from build123d import *

# Parameters (mm, degrees)
SKETCH2_W               = 1500
SKETCH2_H               = 150
BOSS_EXTRUDE1_DEPTH     = 600
SKETCH3_R               = 12.5
CUT_EXTRUDE2_DEPTH      = 250
MIRROR3_COPY_1_SKETCH_R = 12.5
MIRROR3_COPY_1_DEPTH    = 250
SKETCH4_R               = 12.5
CUT_EXTRUDE3_DEPTH      = 50
SKETCH5_W               = 1020
SKETCH5_H               = 1050
CUT_EXTRUDE4_DEPTH      = 100
FILLET1_R               = 20


with BuildPart() as part:
    # Sketch2 → Boss-Extrude1 (new body, symmetric)
    with BuildSketch(Plane.XY):
        Rectangle(SKETCH2_W, SKETCH2_H)
    extrude(amount=BOSS_EXTRUDE1_DEPTH, both=True)

    # Sketch3 → Cut-Extrude2 (cut)
    with BuildSketch(Plane.XY.offset(600)):
        with Locations((-600, -25)):
            Circle(SKETCH3_R)
    cut_extrude2 = extrude(amount=-CUT_EXTRUDE2_DEPTH, mode=Mode.SUBTRACT)

    # Mirror2: Cut-Extrude2 across plane
    add(cut_extrude2.mirror(Plane(origin=(0, 0, 0), x_dir=(0, 0, 1), z_dir=(1, 0, 0))), mode=Mode.SUBTRACT)

    # Mirror3: Cut-Extrude2 across plane
    add(cut_extrude2.mirror(Plane.XY), mode=Mode.SUBTRACT)

    # Mirror3 copy 1 sketch → Mirror3 copy 1 (cut)
    with BuildSketch(Plane(origin=(0, 0, -600), x_dir=(-1, 0, 0), z_dir=(0, 0, -1))):
        with Locations((-600, -25)):
            Circle(MIRROR3_COPY_1_SKETCH_R)
    extrude(amount=-MIRROR3_COPY_1_DEPTH, mode=Mode.SUBTRACT)

    # Sketch4 → Cut-Extrude3 (cut)
    with BuildSketch(Plane(origin=(0, 75, 0), x_dir=(1, 0, 0), z_dir=(0, 1, 0))):
        with Locations((-650, 0)):
            Circle(SKETCH4_R)
    extrude(amount=-CUT_EXTRUDE3_DEPTH, mode=Mode.SUBTRACT)

    # Sketch5 → Cut-Extrude4 (cut)
    with BuildSketch(Plane(origin=(0, 75, 0), x_dir=(1, 0, 0), z_dir=(0, 1, 0))):
        Rectangle(SKETCH5_W, SKETCH5_H)
    extrude(amount=-CUT_EXTRUDE4_DEPTH, mode=Mode.SUBTRACT)

    # Fillet1
    fillet1_edges = [part.edges().sort_by_distance(p)[0] for p in [
        (-750, 0, 600),
        (0, -75, 600),
        (510, -25, 0),
        (510, 25, -525),
        (0, -25, 525),
        (510, 25, 525),
        (-510, -25, 0),
        (-510, 25, 525),
        (0, -25, -525),
        (-510, 25, -525),
        (510, 75, 0),
        (0, 75, -525),
        (-510, 75, 0),
        (0, 75, 525),
        (750, 0, 600),
        (0, -75, -600),
        (-750, 0, -600),
        (750, 0, -600),
        (750, -75, 0),
        (-750, -75, 0),
    ]]
    fillet(fillet1_edges, radius=FILLET1_R)


solid = part.part
Can you work these out from the model? Positions are in its coordinate system, mm. A direction names the side the tool comes from. Coordinates: 2 decimals unless noted, no trailing zeros. Write each loop counter-clockwise with the first axis right and the second up, starting at its lowest first coordinate (ties: lowest second). Pieces come first, ordered by that corner, then holes. Notation, with made-up numbers: (87, 80) -> (99, 80) arc R7 ccw to (99, 92) -> close; hole circle Ø7 at (17, -37). An arc over 180 degrees is marked (long way). Answer as CSV lines item,"result".
1) On a 3-axis mill with a long thin cutter (end or side, diameter ignored), from which of +Z, -Z, +X, -X, +Y, -Y can I reach the whole of each face in a straight line? I mean faces 5 (the flat face through (-10, 11, -600)), 6 (the flat face through (510, 25, 7)). Say none if no direction works.
Check result:
face 5,"-Z, +X, -X, +Y, -Y"
face 6,"+Y"
2) If we section it at B-B on x = -189: Please give me the cut outline in (y, z).
Check result:
outline,"(-75, -580) arc R20 ccw to (-55, -600) -> (75, -600) -> (75, -545) arc R20 ccw to (55, -525) -> (-5, -525) arc R20 cw to (-25, -505) -> (-25, 505) arc R20 cw to (-5, 525) -> (55, 525) arc R20 ccw to (75, 545) -> (75, 600) -> (-55, 600) arc R20 ccw to (-75, 580) -> close"
3) If we mould it in two halves opening along X, with no side actions, what happens to faces 1 (the flat face through (-510, 25, 7)), 2 (the flat face through (-7, 25, -525)), 3 (the flat face through (-10, -75, 8)), 4 (the flat face through (750, 9, 8))? For each: +X half, -X half, draft (parallel to the pull), parting line (faces both ways), or undercut.
Check result:
face 1,"undercut"
face 2,"undercut"
face 3,"draft"
face 4,"+X half"
4) Will these pins go through, and if not, where does the flat tip stop? P1, Ø7.5, axis at x = -601, y = -27, coming from the +Z side; P2, Ø12, axis at x = 244, z = 363.5, coming from the +Y side; P3, Ø15, axis at x = 600, y = -25, coming from the -Z side.
Check result:
P1,"z = 350"
P2,"y = -25"
P3,"z = -350"
5) If we section it at A-A on z = -369.5: Please give me the cut outline in (x, y), then the cut area to 3 significant figures.
Check result:
outline,"(-750, -55) arc R20 ccw to (-730, -75) -> (730, -75) arc R20 ccw to (750, -55) -> (750, 75) -> (530, 75) arc R20 ccw to (510, 55) -> (510, -5) arc R20 cw to (490, -25) -> (-490, -25) arc R20 cw to (-510, -5) -> (-510, 55) arc R20 ccw to (-530, 75) -> (-750, 75) -> close; hole circle Ø25 at (-600, -25); hole circle Ø25 at (600, -25)"
area,"122,000 mm²"
6) If we section it at C-C on z = -77.5: Please give me the cut outline in (x, y), then the cut area to 3 significant figures.
Check result:
outline,"(-750, -55) arc R20 ccw to (-730, -75) -> (730, -75) arc R20 ccw to (750, -55) -> (750, 75) -> (530, 75) arc R20 ccw to (510, 55) -> (510, -5) arc R20 cw to (490, -25) -> (-490, -25) arc R20 cw to (-510, -5) -> (-510, 55) arc R20 ccw to (-530, 75) -> (-750, 75) -> close"
area,"123,000 mm²"
7) If I drill on line 1 (X direction, y = 53, z = 0); line 2 (Z direction, x = -650, y = 49); line 3 (Y direction, x = -600, z = 488), over which ranges is the centre line in solid material (lowest first)? Write a range as from..to.
Check result:
line 1,"-750..-662.5, -637.5..-510, 510..750"
line 2,"-600..-12.5, 12.5..600"
line 3,"-75..-37.5, -12.5..75"
